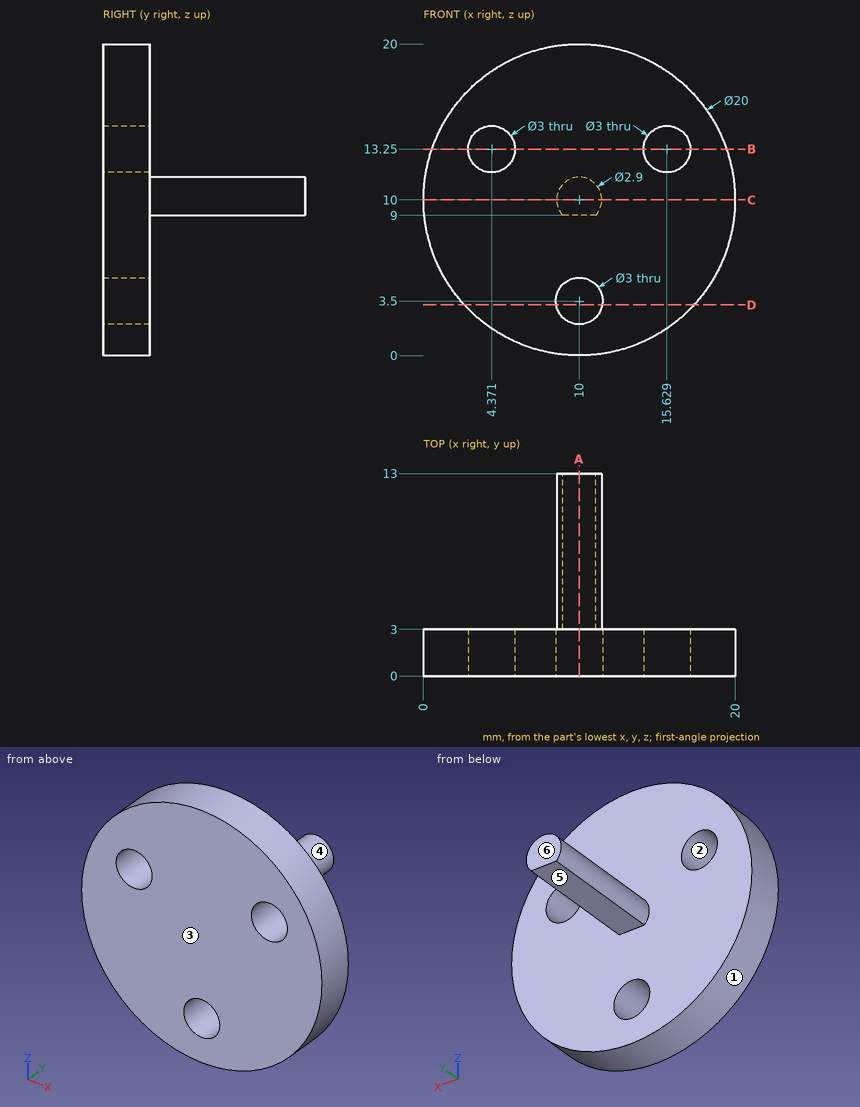
Can you work these out from the drawing? Everything is in mm from the part's minimum corner. A direction names the side the tool comes from. Round coordinates to 2 decimals unless told otherwise and drop trailing zeros. Write each loop counter-clockwise with the first axis right and the second up, starting at its lowest first coordinate (ties: lowest second). Pieces come first, ordered by that corner, then holes. Notation, with made-up numbers: (53.25, 85) - (80.25, 85) arc R27 cw to (80.25, 112) - close; hole circle Ø5 at (48.25, 30). An arc over 180 degrees is marked (long way). Write each question's results on one line, items separated by ' | '. Start each with the question number.
1) Suppose I cut it at D-D (z = 3.25). List the corners of the cut face in (x, y) for me, and give its area (3 significant figures).
2) Suppose I cut it at B-B (z = 13.25). List the corners of the cut face in (x, y) for me.
3) For pin 1 Ø3 at (x, z) = (8, 9) entering from +Y; pin 2 Ø4 at (x, y) = (12, 7) entering from -Z; pin 3 Ø6 at (x, y) = (14.5, 5) entering from -Z; pin 4 Ø3.5 at (x, z) = (15.63, 13.25) entering from +Y, each with a flat end and sliding along its axis, tell me the tip position at first contact or that it passes through.
4) Suppose I cut it at A-A (x = 10). List the corners of the cut face in (y, z) for me.
5) Please list where these lines run through material, in increasing order: line 1 (Y direction, x = 6.25, z = 12); line 2 (X direction, y = 2.05, z = 13.25); line 3 (X direction, y = 6.5, z = 10).
6) Which directions (+Z, -Z, +X, -X, +Y, -Y) give clear straight access to the entire face, cutting with the end or side of a thin tool? Please do the marked faces 4, 5 and 6.
7) Suppose I cut it at C-C (z = 10). List the corners of the cut face in (x, y) for me, and give its area (3 significant figures).
8) We'd pull the mould along X, two halves only. Please class the marked faces 1, 2 and 3: released by +X, released by -X, zero draft, split by the parting line, or undercut.
Here are the results:
1) outline: (2.62, 0) - (8.52, 0) - (8.52, 3) - (2.62, 3) - close; (11.48, 0) - (17.38, 0) - (17.38, 3) - (11.48, 3) - close | area: 35.4 mm2
2) outline: (0.54, 0) - (2.87, 0) - (2.87, 3) - (0.54, 3) - close; (5.87, 0) - (14.13, 0) - (14.13, 3) - (5.87, 3) - close; (17.13, 0) - (19.46, 0) - (19.46, 3) - (17.13, 3) - close
3) pin 1: stops at y = 13 | pin 2: stops at z = 9 | pin 3: stops at z = 0.26 | pin 4: stops at y = 3
4) outline: (0, 0) - (3, 0) - (3, 2) - (0, 2) - close; (0, 5) - (3, 5) - (3, 9) - (13, 9) - (13, 11.45) - (3, 11.45) - (3, 20) - (0, 20) - close
5) line 1: y = 0 to 3 | line 2: x = 0.54 to 2.87, 5.87 to 14.13, 17.13 to 19.46 | line 3: x = 8.55 to 11.45
6) face 4: +Y | face 5: -Z, +X, -X, +Y | face 6: +Z, -Z, +X, -X, +Y
7) outline: (0, 0) - (20, 0) - (20, 3) - (11.45, 3) - (11.45, 13) - (8.55, 13) - (8.55, 3) - (0, 3) - close | area: 89.0 mm2
8) face 1: split by the parting line | face 2: undercut | face 3: zero draft
